```python
from build123d import *

# Parameters (mm, degrees)
SKETCH1_W           = 25
SKETCH1_H           = 21
BOSS_EXTRUDE1_DEPTH = 15
SKETCH2_W           = 15
SKETCH2_H           = 3.4
CUT_EXTRUDE1_DEPTH  = 22.6
CUT_EXTRUDE2_DEPTH  = 5
FILLET1_R           = 1
SKETCH4_W           = 2.4
SKETCH4_H           = 15
CUT_EXTRUDE4_DEPTH  = 64.025788373


with BuildPart() as part:
    # Sketch1 → Boss-Extrude1 (new body)
    with BuildSketch(Plane(origin=(0, 0, 0), x_dir=(1, 0, 0), z_dir=(0, 1, 0))):
        Rectangle(SKETCH1_W, SKETCH1_H)
    extrude(amount=BOSS_EXTRUDE1_DEPTH)

    # Sketch2 → Cut-Extrude1 (cut)
    with BuildSketch(Plane.ZY.offset(12.5)):
        with Locations((-3, 3.7)):
            Rectangle(SKETCH2_W, SKETCH2_H)
    extrude(amount=-CUT_EXTRUDE1_DEPTH, mode=Mode.SUBTRACT)

    # Sketch3 → Cut-Extrude2 (cut)
    with BuildSketch(Plane(origin=(0, 15, 0), x_dir=(1, 0, 0), z_dir=(0, 1, 0))):
        Polygon((-4.85, -0.925), (-4.85, -8.575), (-7.5, -8.575), (-7.5, -6.325), (-12.5, -6.325), (-12.5, -3.175), (-7.5, -3.175), (-7.5, -0.925), align=None)
        Polygon((-3.575, 10.5), (-3.575, 5.5), (-5.825, 5.5), (-5.825, 2.85), (1.825, 2.85), (1.825, 5.5), (-0.425, 5.5), (-0.425, 10.5), align=None)
    extrude(amount=-CUT_EXTRUDE2_DEPTH, mode=Mode.SUBTRACT)

    # Fillet1
    fillet1_edges = [part.edges().sort_by_distance(p)[0] for p in [
        (-6.175, 15, 0.925),
        (-7.5, 15, 2.05),
        (-10, 15, 3.175),
        (-10, 15, 6.325),
        (-7.5, 15, 7.45),
        (-6.175, 15, 8.575),
        (-4.85, 15, 4.75),
        (-3.575, 15, -8),
        (-4.7, 15, -5.5),
        (-5.825, 15, -4.175),
        (-2, 15, -2.85),
        (1.825, 15, -4.175),
        (0.7, 15, -5.5),
        (-0.425, 15, -8),
    ]]
    fillet(fillet1_edges, radius=FILLET1_R)


with BuildPart() as body_2:
    # Mirror2: mirrored copy
    add(part.part.mirror(Plane.ZY.offset(22.5)))

    # Sketch4 → Cut-Extrude4 (cut, through all)
    with BuildSketch(Plane(origin=(0, 0, -10.5), x_dir=(-1, 0, 0), z_dir=(0, 0, -1))):
        with Locations((56.3, 7.5)):
            Rectangle(SKETCH4_W, SKETCH4_H)
    extrude(amount=-CUT_EXTRUDE4_DEPTH, mode=Mode.SUBTRACT)


solid = body_2.part
```
Geometry check sheet. Reference: the model listing, model coordinates, mm. A direction names the side the tool comes from. Coordinates: 2 decimals unless noted, no trailing zeros. Order: outer loops, then holes, each group sorted by start corner. A loop starts at its lowest first (then second) coordinate and runs counter-clockwise, first axis right, second up. Notation, with made-up numbers: (-28, 28.5) - (-24, 28.5) arc R20 ccw to (-24, 58.5) - close; hole circle Ø11 at (24, 48.25). An arc over 180 degrees is marked (long way). Answer as a JSON object with one key per item and string values. Group by question number.
Item 1: Sectioned sample at A-A, the plane z = 4. Record the cut outline in (x, y), and give its area (3 significant figures).
Item 2: Sectioned sample at C-C, the plane y = 13.5. Record the cut outline in (x, z) (3 decimals), and give its area (3 significant figures).
Item 3: Scan lines: probe 1 along Y at (x, z) = (-41.5, 4.25); probe 2 along Z at (x, y) = (-33.5, 12.75) (3 decimals); probe 3 along Z at (x, y) = (-39.75, 14.25). Record each from-to range of solid material in increasing order.
Item 4: Tool access check on faces 5 (the face through (-39, 12, 8.575)), 6 (the face through (-44.876, 14.715, -8.035)), 7 (the face through (-35, 12, 6.325)). Record the directions out of +Z, -Z, +X, -X, +Y, -Y that give a thin tool (end or side, any length) a straight path to the whole face; none if there is none.
Item 5: Sectioned sample at B-B, the plane x = -53. Record the cut outline in (y, z), and give its area (3 significant figures).
Item 6: Draft check along X on faces 1 (the face through (-40.451, 14.715, 4.818)), 2 (the face through (-32.5, 7, 0)), 3 (the face through (-47.26, 14.825, -4.208)), 4 (the face through (-44, 0, 0)). Enter one of: +X half, -X half, draft (parallel to the pull), parting line (faces both ways), or undercut.
Item 7: Sectioned sample at D-D, the plane z = 0.25. Record the cut outline in (x, y) (3 decimals), and give its area (3 significant figures).
Resolved:
{
 "1": {"outline": "(-55.1, 0) - (-32.5, 0) - (-32.5, 2) - (-55.1, 2) - close; (-55.1, 5.4) - (-32.5, 5.4) - (-32.5, 10) - (-40.15, 10) - (-40.15, 14) arc R1 ccw to (-41.15, 15) - (-55.1, 15) - close", "area": "224 mm^2"},
 "2": {"outline": "(-55.1, -10.5) - (-44.575, -10.5) - (-44.575, -5.5) - (-46.825, -5.5) - (-46.825, -2.85) - (-39.175, -2.85) - (-39.175, -5.5) - (-41.425, -5.5) - (-41.425, -10.5) - (-32.5, -10.5) - (-32.5, 3.175) - (-37.5, 3.175) - (-37.5, 0.925) - (-40.15, 0.925) - (-40.15, 8.575) - (-37.5, 8.575) - (-37.5, 6.325) - (-32.5, 6.325) - (-32.5, 10.5) - (-55.1, 10.5) - close", "area": "403 mm^2"},
 "3": {"probe 1": "0 to 2, 5.4 to 15", "probe 2": "-10.5 to 3.175, 6.325 to 10.5", "probe 3": "-10.5 to -5.53, -2.82 to 0.89, 8.61 to 10.5"},
 "4": {"face 5": "+Y", "face 6": "-Z, +Y", "face 7": "+X, +Y"},
 "5": {"outline": "(0, -10.5) - (2, -10.5) - (2, 4.5) - (5.4, 4.5) - (5.4, -10.5) - (15, -10.5) - (15, 10.5) - (0, 10.5) - close", "area": "264 mm^2"},
 "6": {"face 1": "undercut", "face 2": "+X half", "face 3": "undercut", "face 4": "draft"},
 "7": {"outline": "(-55.1, 0) - (-32.5, 0) - (-32.5, 2) - (-55.1, 2) - close; (-55.1, 5.4) - (-32.5, 5.4) - (-32.5, 15) - (-36.5, 15) arc R1 ccw to (-36.825, 14.946) - (-40.825, 14.946) arc R1 ccw to (-41.15, 15) - (-55.1, 15) - close", "area": "262 mm^2"}
}
